from build123d import *

# Parameters (mm, degrees)
BOSS_EXTRUDE1_DEPTH = 40
SKETCH2_R           = 75
BOSS_EXTRUDE2_DEPTH = 688
SKETCH3_R           = 75
BOSS_EXTRUDE3_DEPTH = 1
SKETCH5_R           = 75
CUT_EXTRUDE1_DEPTH  = 25


with BuildPart() as part:
    # Sketch1 → Boss-Extrude1 (new body)
    with BuildSketch(Plane(origin=(0, 0, 0), x_dir=(1, 0, 0), z_dir=(0, 1, 0))):
        with BuildLine():
            Line((0, 0), (450, 0))
            ThreePointArc((450, 0), (565, 115), (450, 230))
            Line((450, 230), (0, 230))
            ThreePointArc((0, 230), (-115, 115), (0, 0))
        make_face()
    boss_extrude1 = extrude(amount=BOSS_EXTRUDE1_DEPTH)

    # Sketch2 → Boss-Extrude2 (add)
    with BuildSketch(Plane(origin=(0, 40, 0), x_dir=(1, 0, 0), z_dir=(0, 1, 0))):
        with Locations(Location((0, 115, 0), (0, 0, 270))):
            Circle(SKETCH2_R)
        with Locations(Location((450, 115, 0), (0, 0, 270))):
            Circle(SKETCH2_R)
    extrude(amount=BOSS_EXTRUDE2_DEPTH)

    # Mirror1: Boss-Extrude1 across plane
    add(boss_extrude1.mirror(Plane.ZX.offset(384)))

    # Sketch3 → Boss-Extrude3 (add)
    with BuildSketch(Plane(origin=(0, 768, 0), x_dir=(1, 0, 0), z_dir=(0, 1, 0))):
        with Locations(Location((225, 115, 0), (0, 0, 270))):
            Circle(SKETCH3_R)
    boss_extrude3 = extrude(amount=BOSS_EXTRUDE3_DEPTH)

    # Mirror2: Boss-Extrude3 across plane
    add(boss_extrude3.mirror(Plane.ZX.offset(384)))

    # Sketch5 → Cut-Extrude1 (cut)
    with BuildSketch(Plane(origin=(0, 769, 0), x_dir=(1, 0, 0), z_dir=(0, 1, 0))):
        with Locations(Location((225, 115, 0), (0, 0, 270))):
            Circle(SKETCH5_R)
    cut_extrude1 = extrude(amount=-CUT_EXTRUDE1_DEPTH, mode=Mode.SUBTRACT)

    # Mirror3: Cut-Extrude1 across plane
    add(cut_extrude1.mirror(Plane.ZX.offset(384)), mode=Mode.SUBTRACT)


solid = part.part
Read the model definition and answer for the solid it produces. Units are mm, in the model's axes. A direction names the side the tool comes from. Give positions to 0.01 mm unless a question says otherwise; leave off trailing zeros. Write each loop counter-clockwise with the first axis right and the second up, starting at its lowest first coordinate (ties: lowest second). Pieces come first, ordered by that corner, then holes. Notation, with made-up numbers: (37.25, 51) - (95.25, 51) arc R22 ccw to (95.25, 60) - close; hole circle Ø1 at (-7.75, 32). An arc over 180 degrees is marked (long way). Answer in a Markdown table with one row per item. Add a question column.
Item 1: Flat-ended cylindrical pins translate along their axes: P1, Ø2, axis at x = 42, y = 356, coming from the +Z side; P2, Ø1.5, axis at x = 441.5, y = 265.5, coming from the +Z side. Find the tip coordinate at first contact, or state that the pin passes through.
Item 2: Section B-B, the plane x = 93 is taken. Write down the section's boundary in (y, z).
Item 3: Find the intervals of material crossed by L1, parallel to Y at x = 424.5, z = -34.5; L2, parallel to Y at x = 221.5, z = -177.5; L3, parallel to X at y = 752, z = -115, in increasing order.
Item 4: Section C-C, the plane y = 403 is taken. Write down the section's boundary in (x, z), and give its area (3 significant figures).
Item 5: Section A-A, the plane z = -115 is taken. Write down the section's boundary in (x, y).
Item 6: Determine the mould class of faces 6 (the face through (145, 768, -117)), 7 (the face through (513.24, 379.18, -74.68)), 8 (the face through (-114.972, 19.72, -117.529)) for opening direction Y: pulls with the +Y half, pulls with the -Y half, needs draft (parallel to the pull), parting line crosses it, or undercut.
Item 7: Section D-D, the plane z = -163.5 is taken. Write down the section's boundary in (x, y), and give its area (3 significant figures).
Item 8: A tool of negligible diameter and unlimited length cuts with its end or side. For faces 1 (the face through (564.972, 19.72, -112.471)), 2 (the face through (226, 24, -116)), 3 (the face through (228, 20, -230)), 4 (the face through (226, 744, -116)), 5 (the face through (220, 728, -117)), from which of +Z, -Z, +X, -X, +Y, -Y can it reach the whole face along a straight path? Write none if from no direction.
Recorded:
| question | item | result |
|---|---|---|
| 1 | P1 | stops at z = -52.2 |
| 1 | P2 | stops at z = -40.4 |
| 2 | outline | (0, -230) - (40, -230) - (40, 0) - (0, 0) - close; (728, -230) - (768, -230) - (768, 0) - (728, 0) - close |
| 3 | L1 | y = 0 to 40, 728 to 768 |
| 3 | L2 | y = 24 to 40, 728 to 744 |
| 3 | L3 | x = -115 to 150, 300 to 565 |
| 4 | outline | circle Ø150 at (0, -115); circle Ø150 at (450, -115) |
| 4 | area | 35,300 mm2 |
| 5 | outline | (-115, 0) - (150, 0) - (150, 24) - (300, 24) - (300, 0) - (565, 0) - (565, 40) - (525, 40) - (525, 728) - (565, 728) - (565, 768) - (300, 768) - (300, 744) - (150, 744) - (150, 768) - (-115, 768) - (-115, 728) - (-75, 728) - (-75, 40) - (-115, 40) - close; hole (75, 40) - (375, 40) - (375, 728) - (75, 728) - close |
| 6 | face 6 | pulls with the +Y half |
| 6 | face 7 | undercut |
| 6 | face 8 | needs draft |
| 7 | outline | (-104.27, 0) - (167.79, 0) - (167.79, 24) - (282.21, 24) - (282.21, 0) - (554.27, 0) - (554.27, 40) - (507.21, 40) - (507.21, 728) - (554.27, 728) - (554.27, 768) - (282.21, 768) - (282.21, 744) - (167.79, 744) - (167.79, 768) - (-104.27, 768) - (-104.27, 728) - (-57.21, 728) - (-57.21, 40) - (-104.27, 40) - close; hole (57.21, 40) - (392.79, 40) - (392.79, 728) - (57.21, 728) - close |
| 7 | area | 205,000 mm2 |
| 8 | face 1 | +X, +Y, -Y |
| 8 | face 2 | -Y |
| 8 | face 3 | -Z, +X, -X, +Y, -Y |
| 8 | face 4 | +Y |
| 8 | face 5 | none |
